Autodesk Inventor part; units mm, degrees
ref_plane "YZ Plane" through (0, 0, 0) normal (1, 0, 0) x (0, 1, 0)
ref_plane "XZ Plane" through (0, 0, 0) normal (0, 1, 0) x (-1, 0, 0)
ref_plane "XY Plane" through (0, 0, 0) normal (0, 0, 1) x (1, 0, 0)
sketch "Sketch1" plane through (0, 0, 0) normal (1, 0, 0) x (0, 1, 0)
  circle A0 centre (0, 0) radius 4.7625
  dimension "d0" = 9.525
extrude "Extrusion1" add sketch "Sketch1" along normal blind 158.75
sketch "Sketch2" plane through (158.75, 0, 0) normal (1, 0, 0) x (0, 0, -1)
  circle A0 centre (0, 0) radius 4.7625
hole "Hole1" at (158.75, 0, 0) direction (-1, 0, 0) diameter 4.3434 depth 19.05 tip angle 118
sketch "Sketch3" plane through (0, 0, 0) normal (-1, 0, 0) x (0, 0, 1)
  circle A0 centre (0, 0) radius 2.1717
hole "Hole2" at (0, 0, 0) direction (1, 0, 0) diameter 4.3434 depth 19.05 tip angle 118
properties part number "STOCK,HOOD,SPACER,10-32,6.25in" material "Aluminum 6061"
Source: CAD feature listing. Evaluate the final solid. Frame: model axes, mm. A direction names the side the tool comes from. Round coordinates to 2 decimals unless told otherwise and drop trailing zeros. Loops run counter-clockwise (first coordinate to the right, second up) from the corner with the lowest first, then second, coordinate; pieces in that order, holes last. Notation, with made-up numbers: M 18.5,69.25 L 37.5,69.25 A31 cw 37.5,103.25 Z; hole C -2,30.5 d7. An arc over 180 degrees is marked long. Use a Markdown table: item, result. Add a question column.
1. Reachability of faces 1 (the cylindrical face through (9.66, 2.12, -0.47)), 2 (the cylindrical face through (149.09, 2.12, 0.47)), 3 (the flat face through (0, 2.05, 1.13)) from +Z, -Z, +X, -X, +Y, -Y: full face, straight path, thin tool, end or side. Return the list, or none.
2. Line query: line 1 (Z direction, x = 14.5, y = 0); line 2 (Y direction, x = 19, z = 2); line 3 (Z direction, x = 31, y = 2.75). Output: solid intervals per line, ascending.
3. Mould query, pull axis Y, two halves, no side actions, for faces 4 (the flat face through (158.75, 2.05, 1.13)), 5 (the cylindrical face through (78.26, -3.78, 2.9)), 6 (the conical face through (20.13, -0.23, -0.3)). Classes: pulls with the +Y half, pulls with the -Y half, needs draft (parallel to the pull), parting line crosses it, or undercut.
4. Contact query for flat-ended pins moving along their axis: P1, Ø3, axis at x = 77, z = -2.5, coming from the -Y side; P2, Ø2.5, axis at y = 0, z = 0, coming from the -X side; P3, Ø4, axis at x = 43.5, y = -3, coming from the -Z side. Output: stop coordinate, or through.
5. Section query A-A on x = 12. Return the cut outline in (y, z) (1 decimal).
6. Section query B-B on x = 102. Return the cut outline in (y, z) (1 decimal), then the cut area to 3 significant figures.
Reported:
| question | item | result |
|---|---|---|
| 1 | face 1 | -X |
| 1 | face 2 | +X |
| 1 | face 3 | +Z, -Z, -X, +Y, -Y |
| 2 | line 1 | z = -4.76 to -2.17, 2.17 to 4.76 |
| 2 | line 2 | y = -4.32 to -0.85, 0.85 to 4.32 |
| 2 | line 3 | z = -3.89 to 3.89 |
| 3 | face 4 | needs draft |
| 3 | face 5 | parting line crosses it |
| 3 | face 6 | undercut |
| 4 | P1 | stops at y = -4.66 |
| 4 | P2 | stops at x = 19.6 |
| 4 | P3 | stops at z = -4.66 |
| 5 | outline | C 0,0 d9.5; hole C 0,0 d4.3 |
| 6 | outline | C 0,0 d9.5 |
| 6 | area | 71.3 mm² |
